Design review of the part built by this model. Coordinates are the model's own, in mm. A direction names the side the tool comes from. Round coordinates to 2 decimals unless told otherwise and drop trailing zeros. Order: outer loops, then holes, each group sorted by start corner. A loop starts at its lowest first (then second) coordinate and runs counter-clockwise, first axis right, second up.
from build123d import *

# Parameters (mm, degrees)
BOSS_EXTRUDE1_DEPTH = 77.5
SKETCH2_R           = 3
CUT_EXTRUDE1_DEPTH  = 10


with BuildPart() as part:
    # Sketch1 → Boss-Extrude1 (new body)
    with BuildSketch(Plane.XY):
        Polygon((0, 32.334319527), (0, 19.834319527), (7, 19.834319527), (10, 16.834319527), (10, 14.834319527), (7.75, 12.584319527), (7.75, 10.584319527), (10, 8.334319527), (10, 5.334319527), (22, 5.334319527), (22, 32.334319527), align=None)
        Polygon((-7, 19.834319527), (0, 19.834319527), (0, 32.334319527), (-22, 32.334319527), (-22, 5.334319527), (-10, 5.334319527), (-10, 8.334319527), (-7.75, 10.584319527), (-7.75, 12.584319527), (-10, 14.834319527), (-10, 16.834319527), align=None)
    extrude(amount=-BOSS_EXTRUDE1_DEPTH)

    # Sketch2 → Cut-Extrude1 (cut)
    with BuildSketch(Plane(origin=(0, 32.334319527, 0), x_dir=(1, 0, 0), z_dir=(0, 1, 0))):
        with Locations(Location((-13, 9, 0), (0, 0, 270))):
            Circle(SKETCH2_R)
        with Locations(Location((-13, 68.5, 0), (0, 0, 270))):
            Circle(SKETCH2_R)
        with Locations(Location((13, 68.5, 0), (0, 0, 90))):
            Circle(SKETCH2_R)
        with Locations(Location((13, 9, 0), (0, 0, 90))):
            Circle(SKETCH2_R)
    extrude(amount=-CUT_EXTRUDE1_DEPTH, mode=Mode.SUBTRACT)


solid = part.part
1) Take a section at A-A on x = -13. Give the boundary of the cut face in (y, z).
Results:
outline: (5.33, -77.5) - (32.33, -77.5) - (32.33, -71.5) - (22.33, -71.5) - (22.33, -65.5) - (32.33, -65.5) - (32.33, -12) - (22.33, -12) - (22.33, -6) - (32.33, -6) - (32.33, 0) - (5.33, 0) - close
2) Take a section at D-D on x = 6. Give the boundary of the cut face in (y, z), plus the area to 3 significant figures.
Results:
outline: (19.83, -77.5) - (32.33, -77.5) - (32.33, 0) - (19.83, 0) - close
area: 969 mm2
3) Take a section at C-C on z = -33. Give the boundary of the cut face in (x, y), plus the area to 3 significant figures.
Results:
outline: (-22, 5.33) - (-10, 5.33) - (-10, 8.33) - (-7.75, 10.58) - (-7.75, 12.58) - (-10, 14.83) - (-10, 16.83) - (-7, 19.83) - (7, 19.83) - (10, 16.83) - (10, 14.83) - (7.75, 12.58) - (7.75, 10.58) - (10, 8.33) - (10, 5.33) - (22, 5.33) - (22, 32.33) - (-22, 32.33) - close
area: 926 mm2
4) Take a section at B-B on z = -68.5. Give the boundary of the cut face in (x, y), plus the area to 3 significant figures.
Results:
outline: (-22, 5.33) - (-10, 5.33) - (-10, 8.33) - (-7.75, 10.58) - (-7.75, 12.58) - (-10, 14.83) - (-10, 16.83) - (-7, 19.83) - (7, 19.83) - (10, 16.83) - (10, 14.83) - (7.75, 12.58) - (7.75, 10.58) - (10, 8.33) - (10, 5.33) - (22, 5.33) - (22, 32.33) - (16, 32.33) - (16, 22.33) - (10, 22.33) - (10, 32.33) - (-10, 32.33) - (-10, 22.33) - (-16, 22.33) - (-16, 32.33) - (-22, 32.33) - close
area: 806 mm2
5) The part is to be moulded in two halves that separate along Z. For faces 1 (the face through (22, 19, -38)), 2 (the face through (0, 22, -77.5)), 3 (the face through (-13, 22.334, -69)), say which applies: released by +Z, released by -Z, zero draft, split by the parting line, or undercut.
Results:
face 1: zero draft
face 2: released by -Z
face 3: undercut
6) To check wall thickness, follow line 1 along X through (y, z) = (30, -68.5); line 2 along Z through (x, y) = (13, 25.5); line 3 along Z through (x, y) = (-11.5, 24.5). State the ranges of each line that lie inside material, in increasing order.
Results:
line 1: x = -22 to -16, -10 to 10, 16 to 22
line 2: z = -77.5 to -71.5, -65.5 to -12, -6 to 0
line 3: z = -77.5 to -71.1, -65.9 to -11.6, -6.4 to 0
7) For faces 4 (the face through (-14.8, 27.4, -70.9)), 5 (the face through (-8.891, 9.444, -38.207)), 6 (the face through (-10, 16, -38)), list the 3-axis set-ups (+Z, -Z, +X, -X, +Y, -Y) from which the entire face can be reached by the end or side of a thin tool; tool diameter is ignored.
Results:
face 4: +Y
face 5: +Z, -Z, -Y
face 6: +Z, -Z
8) Clearance check with flat-ended pins moving along their axes: P1, Ø3, axis at x = 12.5, z = -67.5, coming from the +Y side; P2, Ø7, axis at x = -2.5, z = -38.5, coming from the -Y side. State where each tip first meets the part, or that it passes through.
Results:
P1: stops at y = 22.33
P2: stops at y = 19.83
